from build123d import *

# Parameters (mm, degrees)
SKETCH1_R                = 18
SKETCH1_R_2              = 14.5
BOSS_EXTRUDE1_DEPTH      = 130
FILLET1_R                = 3
BOSS_EXTRUDE2_DEPTH      = 6
SKETCH4_R                = 1.5
CUT_EXTRUDE1_DEPTH       = 1.5
BOSS_EXTRUDE3_DEPTH      = 6
BOSS_EXTRUDE3_DEPTH_BACK = 1
SKETCH5_R                = 3
SKETCH7_R                = 1
CUT_EXTRUDE2_DEPTH       = 6
SKETCH8_R                = 14.5
SKETCH8_R_2              = 11.5
BOSS_EXTRUDE4_DEPTH      = 10
FILLET2_R                = 2


with BuildPart() as part:
    # Sketch1 → Boss-Extrude1 (new body)
    with BuildSketch(Plane(origin=(0, 0, 0), x_dir=(1, 0, 0), z_dir=(0, 1, 0))):
        with Locations(Location((0, 0, 0), (0, 0, 270))):
            Circle(SKETCH1_R)
        with Locations(Location((0, 0, 0), (0, 0, 270))):
            Circle(SKETCH1_R_2, mode=Mode.SUBTRACT)
    extrude(amount=BOSS_EXTRUDE1_DEPTH)

    # Fillet1
    fillet1_edges = [part.edges().sort_by_distance(p)[0] for p in [
        (0, 0, -14.5),
    ]]
    fillet(fillet1_edges, radius=FILLET1_R)

    # Sketch3 → Boss-Extrude2 (add)
    with BuildSketch(Plane(origin=(0, 60, 0), x_dir=(1, 0, 0), z_dir=(0, 1, 0))):
        with BuildLine():
            Line((-3, -19.267848868), (-3, -17.748239349))
            ThreePointArc((-3, -17.748239349), (0, -18), (3, -17.748239349))
            Line((3, -17.748239349), (3, -19.267848868))
            ThreePointArc((3, -19.267848868), (0, -19.5), (-3, -19.267848868))
        make_face()
        with BuildLine():
            Line((3, 19.267848868), (3, 17.748239349))
            ThreePointArc((3, 17.748239349), (0, 18), (-3, 17.748239349))
            Line((-3, 17.748239349), (-3, 19.267848868))
            ThreePointArc((-3, 19.267848868), (0, 19.5), (3, 19.267848868))
        make_face()
    extrude(amount=BOSS_EXTRUDE2_DEPTH)

    # Sketch4 → Cut-Extrude1 (cut, symmetric)
    with BuildSketch(Plane.XY.offset(18)):
        with Locations((0, 63)):
            Circle(SKETCH4_R)
    cut_extrude1 = extrude(amount=CUT_EXTRUDE1_DEPTH, both=True, mode=Mode.SUBTRACT)

    # Mirror1: Cut-Extrude1 across plane
    add(cut_extrude1.mirror(Plane.XY), mode=Mode.SUBTRACT)



with BuildPart() as body_2:
    # Sketch5 → Boss-Extrude3 (new, two sides: drawn at the far end of the back side and taken through both)
    with BuildSketch(Plane.XY.offset(18).offset(-BOSS_EXTRUDE3_DEPTH_BACK)):
        with Locations((0, 13)):
            Circle(SKETCH5_R)
    extrude(amount=BOSS_EXTRUDE3_DEPTH + BOSS_EXTRUDE3_DEPTH_BACK)


with BuildPart() as part_1:
    add(part.part)

    add(body_2.part)  # Revolve1 merges body 2
    # Sketch6 → Revolve1 (revolve)
    with BuildSketch(Plane(origin=(0, 0, 0), x_dir=(0, 0, -1), z_dir=(1, 0, 0)), mode=Mode.PRIVATE) as revolve1_sk:
        with BuildLine():
            Line((-22.744590516, 16), (-22.744590516, 13))
            Line((-22.744590516, 13), (-16.500678741, 13))
            Line((-16.500678741, 13), (-16.500678741, 17.154644063))
            add(Edge.make_bspline(
                [(-16.500678741, 17.154644063), (-18.548555394, 16.616818558), (-20.629859319, 16.231937203), (-22.744590516, 16)],
                knots=[0.47611858, 0.47611858, 0.47611858, 0.47611858, 1, 1, 1, 1], degree=3))
        make_face()
    revolve(revolve1_sk.sketch.rotate(Axis((0, 13, 22.744590516), (0, 0, -1)), 90), axis=Axis((0, 13, 22.744590516), (0, 0, -1)))

    # Sketch7 → Cut-Extrude2 (cut)
    with BuildSketch(Plane.XY.offset(24)):
        with Locations((0, 13)):
            Circle(SKETCH7_R)
    extrude(amount=-CUT_EXTRUDE2_DEPTH, mode=Mode.SUBTRACT)

    # Sketch8 → Boss-Extrude4 (add)
    with BuildSketch(Plane(origin=(0, 70, 0), x_dir=(1, 0, 0), z_dir=(0, 1, 0))):
        with Locations(Location((0, 0, 0), (0, 0, 270))):
            Circle(SKETCH8_R)
        with Locations(Location((0, 0, 0), (0, 0, 270))):
            Circle(SKETCH8_R_2, mode=Mode.SUBTRACT)
    extrude(amount=BOSS_EXTRUDE4_DEPTH)

    # Fillet2
    fillet2_edges = [part_1.edges().sort_by_distance(p)[0] for p in [
        (0, 80, -14.5),
    ]]
    fillet(fillet2_edges, radius=FILLET2_R)


solid = part_1.part
Source: CAD feature listing. Evaluate the final solid. Frame: model axes, mm. A direction names the side the tool comes from. Coordinates: 2 decimals unless noted, no trailing zeros. Order: outer loops, then holes, each group sorted by start corner. A loop starts at its lowest first (then second) coordinate and runs counter-clockwise, first axis right, second up. Notation, with made-up numbers: M 84,-23 L 130,-23 A19 cw 130,14 Z; hole C 39.25,22.5 d11. An arc over 180 degrees is marked long. Write each question's results on one line, items separated by ' | '. Start each with the question number.
1. Pin query (flat end, axial travel): pin 1 (17.5 mm diameter, centred on x = 0, z = 0, fed in from -Y); pin 2 (5 mm diameter, centred on x = 7.5, z = 7, fed in from -Y); pin 3 (0.5 mm diameter, centred on x = 1, z = -18.5, fed in from -Y); pin 4 (5 mm diameter, centred on x = -8.5, y = 17, fed in from +Z). Return the tip coordinate at first contact, or that it passes through.
2. Section B-B, the plane y = 63. Return the cut outline in (x, z), then the cut area to 3 significant figures.
3. Section A-A, the plane y = 87. Return the cut outline in (x, z).
4. Reachability of faces 1 (the face through (-5.554, 105.664, 13.394)), 2 (the face through (8, 70, -9)), 3 (the face through (0, 63, 16.5)), 4 (the face through (0.806, 64.265, -18.021)), 5 (the face through (1.38, 61.62, 19.45)) from +Z, -Z, +X, -X, +Y, -Y: full face, straight path, thin tool, end or side. Return the list, or none.
5. Draft query along Y for faces 6 (the face through (-11, 80, 4)), 7 (the face through (0, 63, -16.5)), 8 (the face through (9.7, 74.93, 6.18)), 9 (the face through (-0.65, 10.07, 23.36)). Return one class per face: +Y half, -Y half, draft (parallel to the pull), parting line (faces both ways), or undercut.
6. Material intervals for L1, parallel to X at y = 108, z = 0; L2, parallel to Y at x = 0, z = 18.3; L3, parallel to X at y = 63, z = 17.9, sorted ascending.
Solution:
1) pin 1: through | pin 2: y = 70 | pin 3: y = 60 | pin 4: z = 16.97
2) outline: M -3,-19.27 A19.5 ccw -1.5,-19.44 L -1.5,-16.5 L 1.5,-16.5 L 1.5,-19.44 A19.5 ccw 3,-19.27 L 3,-17.75 A18 ccw 3,17.75 L 3,19.27 A19.5 ccw 1.5,19.44 L 1.5,16.5 L -1.5,16.5 L -1.5,19.44 A19.5 ccw -3,19.27 L -3,17.75 A18 ccw -3,-17.75 Z; hole C 0,0 d29 | area: 358 mm²
3) outline: C 0,0 d36; hole C 0,0 d29
4) face 1: +Y | face 2: -Y | face 3: +Z | face 4: -Z | face 5: +Z, +Y
5) face 6: +Y half | face 7: undercut | face 8: draft | face 9: parting line
6) L1: -18 to -14.5, 14.5 to 18 | L2: 9.28 to 12, 14 to 16.72, 60 to 61.5, 64.5 to 66 | L3: -3 to -1.5, 1.5 to 3
